```python
from build123d import *

# Parameters (mm, degrees)
SKETCH1_W           = 170
SKETCH1_H           = 57
BOSS_EXTRUDE1_DEPTH = 7
SKETCH2_R           = 10
SKETCH2_R_2         = 3.81
BOSS_EXTRUDE2_DEPTH = 7
FILLET1_R           = 5
FILLET2_R           = 3


with BuildPart() as part:
    # Sketch1 → Boss-Extrude1 (new body)
    with BuildSketch(Plane(origin=(0, 0, 0), x_dir=(1, 0, 0), z_dir=(0, 1, 0))):
        Rectangle(SKETCH1_W, SKETCH1_H)
    extrude(amount=BOSS_EXTRUDE1_DEPTH)

    # Sketch2 → Boss-Extrude2 (add)
    # profile 1 of 8: a face of its own
    with BuildSketch(Plane(origin=(0, 7, 0), x_dir=(1, 0, 0), z_dir=(0, 1, 0))):
        with Locations((-25.4, 36)):
            Circle(SKETCH2_R)
        with Locations(Location((-25.4, 36, 0), (0, 0, 270))):
            Circle(SKETCH2_R_2, mode=Mode.SUBTRACT)
    # profile 2 of 8: a face of its own
    with BuildSketch(Plane(origin=(0, 7, 0), x_dir=(1, 0, 0), z_dir=(0, 1, 0))):
        with Locations((25.4, 36)):
            Circle(SKETCH2_R)
        with Locations(Location((25.4, 36, 0), (0, 0, 270))):
            Circle(SKETCH2_R_2, mode=Mode.SUBTRACT)
    # profile 3 of 8: a face of its own
    with BuildSketch(Plane(origin=(0, 7, 0), x_dir=(1, 0, 0), z_dir=(0, 1, 0))):
        with Locations((-93, 12.7)):
            Circle(SKETCH2_R)
        with Locations(Location((-93, 12.7, 0), (0, 0, 270))):
            Circle(SKETCH2_R_2, mode=Mode.SUBTRACT)
    # profile 4 of 8: a face of its own
    with BuildSketch(Plane(origin=(0, 7, 0), x_dir=(1, 0, 0), z_dir=(0, 1, 0))):
        with Locations((-93, -12.7)):
            Circle(SKETCH2_R)
        with Locations(Location((-93, -12.7, 0), (0, 0, 270))):
            Circle(SKETCH2_R_2, mode=Mode.SUBTRACT)
    # profile 5 of 8: a face of its own
    with BuildSketch(Plane(origin=(0, 7, 0), x_dir=(1, 0, 0), z_dir=(0, 1, 0))):
        with Locations((93, -12.7)):
            Circle(SKETCH2_R)
        with Locations(Location((93, -12.7, 0), (0, 0, 270))):
            Circle(SKETCH2_R_2, mode=Mode.SUBTRACT)
    # profile 6 of 8: a face of its own
    with BuildSketch(Plane(origin=(0, 7, 0), x_dir=(1, 0, 0), z_dir=(0, 1, 0))):
        with Locations((93, 12.7)):
            Circle(SKETCH2_R)
        with Locations(Location((93, 12.7, 0), (0, 0, 270))):
            Circle(SKETCH2_R_2, mode=Mode.SUBTRACT)
    # profile 7 of 8: a face of its own
    with BuildSketch(Plane(origin=(0, 7, 0), x_dir=(1, 0, 0), z_dir=(0, 1, 0))):
        with Locations((25.4, -36)):
            Circle(SKETCH2_R)
        with Locations(Location((25.4, -36, 0), (0, 0, 270))):
            Circle(SKETCH2_R_2, mode=Mode.SUBTRACT)
    # profile 8 of 8: a face of its own
    with BuildSketch(Plane(origin=(0, 7, 0), x_dir=(1, 0, 0), z_dir=(0, 1, 0))):
        with Locations((-25.4, -36)):
            Circle(SKETCH2_R)
        with Locations(Location((-25.4, -36, 0), (0, 0, 270))):
            Circle(SKETCH2_R_2, mode=Mode.SUBTRACT)
    extrude(amount=-BOSS_EXTRUDE2_DEPTH)

    # Fillet1
    # the kernel refuses this fillet: 5 mm, written as the material it adds along each edge
    with BuildSketch(Plane(origin=(-18.785621722, 0, -28.5), x_dir=(1, 0, 0), z_dir=(0, 1, 0)), Plane(origin=(32.014378278, 0, -28.5), x_dir=(1, 0, 0), z_dir=(0, 1, 0)), Plane(origin=(18.785621722, 0, 28.5), x_dir=(-1, 0, 0), z_dir=(0, 1, 0)), Plane(origin=(-32.014378278, 0, 28.5), x_dir=(-1, 0, 0), z_dir=(0, 1, 0))) as fillet1_piece_1:
        with BuildLine():
            CenterArc((8.17582118, 5), FILLET1_R, 170.405931773, 99.594068227)
            ThreePointArc((3.245754694, 5.833333333), (2.124003991, 2.63783224), (0, 0))
            Line((0, 0), (8.17582118, 0))
        make_face()
    extrude(amount=7)
    with BuildSketch(Plane(origin=(-32.014378278, 0, -28.5), x_dir=(-1, 0, 0), z_dir=(0, 1, 0))) as fillet1_piece_2:
        with BuildLine():
            CenterArc((8.17582118, -5), FILLET1_R, 90, 99.594068227)
            ThreePointArc((3.245754694, -5.833333333), (2.124003991, -2.63783224), (0, 0))
            Line((0, 0), (8.17582118, 0))
        make_face()
    extrude(amount=7)
    with BuildSketch(Plane(origin=(18.785621722, 0, -28.5), x_dir=(-0.4862167760179408, 0, -0.8738382268582209), z_dir=(0, 1, 0)), Plane(origin=(32.014378278, 0, 28.5), x_dir=(0.4862167760179433, 0, 0.8738382268582195), z_dir=(0, 1, 0)), Plane(origin=(-18.785621722, 0, 28.5), x_dir=(0.4862167760179409, 0, 0.8738382268582208), z_dir=(0, 1, 0))) as fillet1_piece_3:
        with BuildLine():
            CenterArc((8.34441255, 4.713261203), FILLET1_R, 150.907776941, 99.594068227)
            Line((3.975221415, 7.144345083), (0, 0))
            ThreePointArc((0, 0), (3.33776502, 0.573477594), (6.67553004, 0))
        make_face()
    extrude(amount=7)
    with BuildSketch(Plane(origin=(-85, 0, -18.7), x_dir=(0, 0, -1), z_dir=(0, 1, 0)), Plane(origin=(-85, 0, 6.7), x_dir=(0, 0, -1), z_dir=(0, 1, 0)), Plane(origin=(85, 0, 18.7), x_dir=(0, 0, 1), z_dir=(0, 1, 0)), Plane(origin=(85, 0, -6.7), x_dir=(0, 0, 1), z_dir=(0, 1, 0))) as fillet1_piece_4:
        with BuildLine():
            CenterArc((8.696938457, 5), FILLET1_R, 168.463040967, 101.536959033)
            ThreePointArc((3.797958971, 6), (2.449489743, 2.651530772), (0, 0))
            Line((0, 0), (8.696938457, 0))
        make_face()
    extrude(amount=7)
    with BuildSketch(Plane(origin=(-85, 0, -6.7), x_dir=(-0.8449489742783158, 0, 0.5348469228349566), z_dir=(0, 1, 0)), Plane(origin=(-85, 0, 18.7), x_dir=(-0.844948974278316, 0, 0.5348469228349564), z_dir=(0, 1, 0)), Plane(origin=(85, 0, 6.7), x_dir=(0.8449489742783187, 0, -0.5348469228349522), z_dir=(0, 1, 0)), Plane(origin=(85, 0, -18.7), x_dir=(0.8449489742783186, 0, -0.5348469228349523), z_dir=(0, 1, 0))) as fillet1_piece_5:
        with BuildLine():
            CenterArc((8.876275643, 4.674234614), FILLET1_R, 147.666469307, 101.536959033)
            Line((4.651530772, 7.348469228), (0, 0))
            ThreePointArc((0, 0), (3.550510257, 0.651530772), (7.101020514, 0))
        make_face()
    extrude(amount=7)

    # Fillet2
    # the kernel refuses this fillet: 3 mm, written as the material it adds along each edge
    with BuildSketch(Plane(origin=(-85.416089355, 7, 0), x_dir=(-0.8209960620456767, 0, 0.5709338544047737), z_dir=(0, -1, 0)), Plane(origin=(85.416089355, 7, 0), x_dir=(0.8209960620456767, 0, -0.5709338544047737), z_dir=(0, -1, 0))) as fillet2_piece_1:
        with BuildLine():
            CenterArc((3.672553945, 2.553953029), FILLET2_R, 127.986021581, 173.658700766)
            ThreePointArc((1.826146326, 4.918435827), (0.216147897, 2.717976503), (0, 0))
            ThreePointArc((0, 0), (2.623252818, -0.743411618), (5.246505636, 0))
        make_face()
    extrude(amount=7)


solid = part.part
```
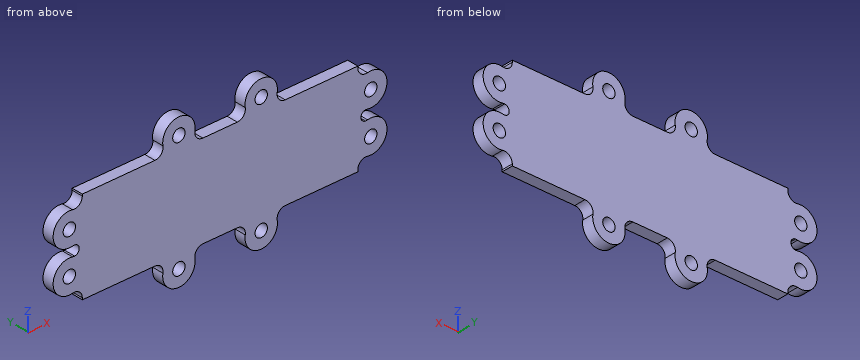
Part model, mm, in its own coordinate system. Give positions to 0.01 mm unless a question says otherwise; leave off trailing zeros. Order: outer loops, then holes, each group sorted by start corner. A loop starts at its lowest first (then second) coordinate and runs counter-clockwise, first axis right, second up. Notation, with made-up numbers: M 83.25,34.5 L 117.25,34.5 A11 cw 117.25,42.5 Z; hole C -32,59 d10. An arc over 180 degrees is marked long. Use a Markdown table: item, result. Add a question column.
(1) Probe line 1 along X through (y, z) = (3.5, 36); line 2 along X through (y, z) = (3.75, 12.7); line 3 along X through (y, z) = (5.5, 37). List the from-to ranges inside material, lowest first. Write a range as [from, to].
(2) Saw through at B-B, the plane z = -12.7. Give the cut face in (x, y), and give its area (3 significant figures).
(3) Saw through at C-C, the plane x = 25.4. Give the cut face in (y, z).
(4) Saw through at D-D, the plane z = 0. Give the cut face in (x, y).
(5) Saw through at A-A, the plane x = -93. Give the cut face in (y, z), and give its area (3 significant figures).
(6) Drop flat-ended pins along their axis: P1, Ø0.9, axis at y = 2.5, z = 28, coming from the -X side; P2, Ø3, axis at x = -50, y = 4, coming from the +Z side; P3, Ø10, axis at x = 93, z = -12.7, coming from the -Y side; P4, Ø4.5, axis at x = -25.4, z = -36, coming from the -Y side. Give the stop position or say it passes through.
Answer key:
| question | item | result |
|---|---|---|
| 1 | line 1 | [-35.4, -29.21], [-21.59, -15.4], [15.4, 21.59], [29.21, 35.4] |
| 1 | line 2 | [-103, -96.81], [-89.19, 89.19], [96.81, 103] |
| 1 | line 3 | [-35.35, -29.08], [-21.72, -15.45], [15.45, 21.72], [29.08, 35.35] |
| 2 | outline | M -103,0 L -96.81,0 L -96.81,7 L -103,7 Z; M -89.19,0 L 89.19,0 L 89.19,7 L -89.19,7 Z; M 96.81,0 L 103,0 L 103,7 L 96.81,7 Z |
| 2 | area | 1,340 mm^2 |
| 3 | outline | M 0,-46 L 7,-46 L 7,-39.81 L 0,-39.81 Z; M 0,-32.19 L 7,-32.19 L 7,32.19 L 0,32.19 Z; M 0,39.81 L 7,39.81 L 7,46 L 0,46 Z |
| 4 | outline | M -86.89,0 L 86.89,0 L 86.89,7 L -86.89,7 Z |
| 5 | outline | M 0,-22.7 L 7,-22.7 L 7,-16.51 L 0,-16.51 Z; M 0,-8.89 L 7,-8.89 L 7,-2.7 L 0,-2.7 Z; M 0,2.7 L 7,2.7 L 7,8.89 L 0,8.89 Z; M 0,16.51 L 7,16.51 L 7,22.7 L 0,22.7 Z |
| 5 | area | 173 mm^2 |
| 6 | P1 | x = -85 |
| 6 | P2 | z = 28.5 |
| 6 | P3 | y = 0 |
| 6 | P4 | through |
